Design review of the part built by this model. Coordinates are the model's own, in mm. Face numbers are marked on the shaded views. Give positions to 0.01 mm unless a question says otherwise; leave off trailing zeros. Loops run counter-clockwise (first coordinate to the right, second up) from the corner with the lowest first, then second, coordinate; pieces in that order, holes last. Notation, with made-up numbers: (83.25, 69.25) - (92.25, 69.25) arc R30 cw to (92.25, 97.25) - close; hole circle Ø10 at (-1.75, -25.5). An arc over 180 degrees is marked (long way). Write each question's results on one line, items separated by ' | '.
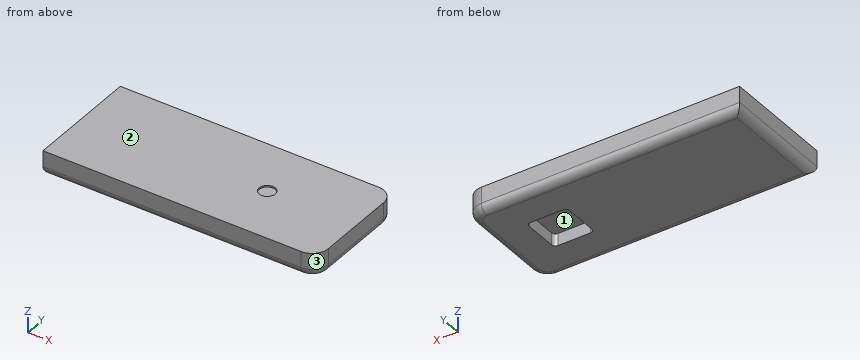
```python
from build123d import *

# Parameters (mm, degrees)
F0_W     = 177.8
F0_H     = 177.8
F1_DEPTH = 38.1
F2_W     = 177.8
F2_H     = 38.1
F3_DEPTH = 254
F4_R     = 25.4
F5_R     = 12.7
F7_DEPTH = 19.05
F8_R     = 12.7
F9_DEPTH = 2.54


with BuildPart() as f1:
    # F0 (on Top) → F1 (new body)
    with BuildSketch(Plane.XY):
        Rectangle(F0_W, F0_H)
    extrude(amount=-F1_DEPTH)

    # F2 (on face) → F3 (join)
    with BuildSketch(Plane(origin=(-88.9, 0, 0), x_dir=(0, -1, 0), z_dir=(-1, 0, 0))):
        with Locations((0, -19.05)):
            Rectangle(F2_W, F2_H)
    extrude(amount=F3_DEPTH)

    # F4
    f4_edges = [f1.edges().sort_by_distance(p)[0] for p in [
        (88.9, 88.9, -19.05),
        (88.9, -88.9, -19.05),
    ]]
    fillet(f4_edges, radius=F4_R)

    # F5
    f5_edges = [f1.edges().sort_by_distance(p)[0] for p in [
        (-139.7, -88.9, -38.1),
        (-342.9, 0, -38.1),
        (-139.7, 88.9, -38.1),
        (81.460512, 81.460512, -38.1),
        (88.9, 0, -38.1),
        (81.460512, -81.460512, -38.1),
    ]]
    fillet(f5_edges, radius=F5_R)

    # F6 (on face) → F7 (cut)
    with BuildSketch(Plane(origin=(0, 0, -38.1), x_dir=(1, 0, 0), z_dir=(0, 0, -1))):
        with BuildLine():
            Line((-25.4, -31.75), (25.4, -31.75))
            ThreePointArc((25.4, -31.75), (29.8901280605, -29.8901280605), (31.75, -25.4))
            Line((31.75, -25.4), (31.75, 25.4))
            ThreePointArc((31.75, 25.4), (29.8901280605, 29.8901280605), (25.4, 31.75))
            Line((25.4, 31.75), (-25.4, 31.75))
            ThreePointArc((-25.4, 31.75), (-29.8901280605, 29.8901280605), (-31.75, 25.4))
            Line((-31.75, 25.4), (-31.75, -25.4))
            ThreePointArc((-31.75, -25.4), (-29.8901280605, -29.8901280605), (-25.4, -31.75))
        make_face()
    extrude(amount=-F7_DEPTH, mode=Mode.SUBTRACT)

    # F8 (on face) → F9 (cut)
    with BuildSketch(Plane.XY):
        with Locations((-50.8, 0)):
            Circle(F8_R)
    extrude(amount=-F9_DEPTH, mode=Mode.SUBTRACT)


solid = f1.part
```
Item 1: We need section A-A on x = 18. Give the boundary of the cut face in (y, z), then the cut area to 3 significant figures.
Output values:
outline: (-88.9, -25.4) arc R12.7 ccw to (-76.2, -38.1) - (-31.75, -38.1) - (-31.75, -19.05) - (31.75, -19.05) - (31.75, -38.1) - (76.2, -38.1) arc R12.7 ccw to (88.9, -25.4) - (88.9, 0) - (-88.9, 0) - close | area: 5,500 mm²
Item 2: Draft analysis for pull direction X (two halves, no side actions). For the marked faces 1, 2 and 3, state which applies: +X half, -X half, draft (parallel to the pull), parting line (faces both ways), or undercut.
Output values:
face 1: undercut | face 2: draft | face 3: +X half
Item 3: We need section C-C on x = -50.8. Give the boundary of the cut face in (y, z), then the cut area to 3 significant figures.
Output values:
outline: (-88.9, -25.4) arc R12.7 ccw to (-76.2, -38.1) - (76.2, -38.1) arc R12.7 ccw to (88.9, -25.4) - (88.9, 0) - (12.7, 0) - (12.7, -2.54) - (-12.7, -2.54) - (-12.7, 0) - (-88.9, 0) - close | area: 6,640 mm²
Item 4: Clearance check with flat-ended pins moving along their axes: P1, Ø9.5, axis at x = 3, z = -33, coming from the -Y side; P2, Ø5.5, axis at y = 11, z = -32, coming from the -X side. State where each tip first meets the part, or that it passes through.
Output values:
P1: stops at y = -88.58 | P2: stops at x = -342.3
Item 5: Wall thickness on probe 1 along Y at (x, z) = (-50.8, -1.85); probe 2 along X at (y, z) = (26, -25.5); probe 3 along Y at (x, z) = (-27, -22): over which ranges is each line inside the solid? List them lowest first.
Output values:
probe 1: y = -88.9 to -12.7, 12.7 to 88.9 | probe 2: x = -342.9 to -31.72, 31.72 to 88.9 | probe 3: y = -88.9 to -31.55, 31.55 to 88.9
Item 6: We need section B-B on y = 0. Give the boundary of the cut face in (x, z).
Output values:
outline: (-342.9, -25.4) arc R12.7 ccw to (-330.2, -38.1) - (-31.75, -38.1) - (-31.75, -19.05) - (31.75, -19.05) - (31.75, -38.1) - (76.2, -38.1) arc R12.7 ccw to (88.9, -25.4) - (88.9, 0) - (-38.1, 0) - (-38.1, -2.54) - (-63.5, -2.54) - (-63.5, 0) - (-342.9, 0) - close
